Check sheet for the modelled part. Datum: model origin and axes. Units: mm. Round coordinates to 2 decimals unless told otherwise and drop trailing zeros. Order: outer loops, then holes, each group sorted by start corner. A loop starts at its lowest first (then second) coordinate and runs counter-clockwise, first axis right, second up.
Q1. Cross-section at C-C on y = 5. Record the cut outline in (x, z).
Q2. Cross-section at D-D on z = 0.55. Give the number of separate pieces and of enclosed holes in the cut face, then the cut area to 3 significant figures.
Q3. Depth check by flat-ended pin: P1, Ø2.5, axis at x = -53.03, y = -53.03, coming from the +Z side. Enter the tip coordinate at first touch or a pass-through.
Q4. Cross-section at A-A on x = 0. Record the cut outline in (y, z), then the cut area to 3 significant figures.
Q5. Cross-section at B-B on y = -23. Record the cut outline in (x, z), then the cut area to 3 significant figures.
Q6. Scan lines: probe 1 along X at (y, z) = (-43, 0.8); probe 2 along Y at (x, z) = (53, 2.3); probe 3 along Y at (x, z) = (-17, 2.3). Record each from-to range of solid material in increasing order.
from build123d import *

# Parameters (mm, degrees)
SKETCH_1_W      = 140
SKETCH_1_H      = 140
SKETCH_1_R      = 1.6
SKETCH_1_R_2    = 1.1
SKETCH_1_R_3    = 15
EXTRUDE_1_DEPTH = 3
FILLET_1_R      = 5


with BuildPart() as part:
    # 草图1 → 凸台-拉伸1 (new body)
    with BuildSketch(Plane.XY):
        Rectangle(SKETCH_1_W, SKETCH_1_H)
        with Locations((53.033008589, 53.033008589)):
            Circle(SKETCH_1_R, mode=Mode.SUBTRACT)
        with Locations((-29, 43)):
            Circle(SKETCH_1_R_2, mode=Mode.SUBTRACT)
        with Locations((29, 43)):
            Circle(SKETCH_1_R_2, mode=Mode.SUBTRACT)
        with Locations(Location((29, -43, 0), (0, 0, 180))):
            Circle(SKETCH_1_R_2, mode=Mode.SUBTRACT)
        with Locations(Location((-29, -43, 0), (0, 0, 180))):
            Circle(SKETCH_1_R_2, mode=Mode.SUBTRACT)
        with Locations((53.033008589, -53.033008589)):
            Circle(SKETCH_1_R, mode=Mode.SUBTRACT)
        with Locations((-53.033008589, -53.033008589)):
            Circle(SKETCH_1_R, mode=Mode.SUBTRACT)
        with Locations((-53.033008589, 53.033008589)):
            Circle(SKETCH_1_R, mode=Mode.SUBTRACT)
        with Locations((45.961940777, 45.961940777)):
            Circle(SKETCH_1_R, mode=Mode.SUBTRACT)
        with Locations((38.890872965, 38.890872965)):
            Circle(SKETCH_1_R, mode=Mode.SUBTRACT)
        with Locations((45.961940777, -45.961940777)):
            Circle(SKETCH_1_R, mode=Mode.SUBTRACT)
        with Locations((38.890872965, -38.890872965)):
            Circle(SKETCH_1_R, mode=Mode.SUBTRACT)
        with Locations((-45.961940777, -45.961940777)):
            Circle(SKETCH_1_R, mode=Mode.SUBTRACT)
        with Locations((-38.890872965, -38.890872965)):
            Circle(SKETCH_1_R, mode=Mode.SUBTRACT)
        with Locations((-45.961940777, 45.961940777)):
            Circle(SKETCH_1_R, mode=Mode.SUBTRACT)
        with Locations((-38.890872965, 38.890872965)):
            Circle(SKETCH_1_R, mode=Mode.SUBTRACT)
        Circle(SKETCH_1_R_3, mode=Mode.SUBTRACT)
        with BuildLine():
            Line((-25, 58.033008589), (25, 58.033008589))
            ThreePointArc((25, 58.033008589), (30, 53.033008589), (25, 48.033008589))
            Line((25, 48.033008589), (-25, 48.033008589))
            ThreePointArc((-25, 48.033008589), (-30, 53.033008589), (-25, 58.033008589))
        make_face(mode=Mode.SUBTRACT)
        with BuildLine():
            Line((58.033008589, 25), (58.033008589, -25))
            ThreePointArc((58.033008589, -25), (53.033008589, -30), (48.033008589, -25))
            Line((48.033008589, -25), (48.033008589, 25))
            ThreePointArc((48.033008589, 25), (53.033008589, 30), (58.033008589, 25))
        make_face(mode=Mode.SUBTRACT)
        with BuildLine():
            Line((25, -58.033008589), (-25, -58.033008589))
            ThreePointArc((-25, -58.033008589), (-30, -53.033008589), (-25, -48.033008589))
            Line((-25, -48.033008589), (25, -48.033008589))
            ThreePointArc((25, -48.033008589), (30, -53.033008589), (25, -58.033008589))
        make_face(mode=Mode.SUBTRACT)
        with BuildLine():
            Line((-58.033008589, -25), (-58.033008589, 25))
            ThreePointArc((-58.033008589, 25), (-53.033008589, 30), (-48.033008589, 25))
            Line((-48.033008589, 25), (-48.033008589, -25))
            ThreePointArc((-48.033008589, -25), (-53.033008589, -30), (-58.033008589, -25))
        make_face(mode=Mode.SUBTRACT)
    extrude(amount=EXTRUDE_1_DEPTH)

    # 圆角1
    fillet_1_edges = [part.edges().sort_by_distance(p)[0] for p in [
        (-70, 70, 1.5),
        (70, 70, 1.5),
        (70, -70, 1.5),
        (-70, -70, 1.5),
    ]]
    fillet(fillet_1_edges, radius=FILLET_1_R)


solid = part.part
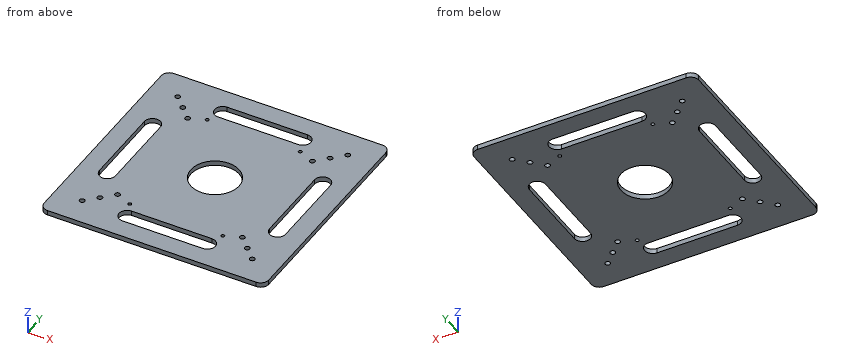
Results found:
1. outline: (-70, 0) - (-58.03, 0) - (-58.03, 3) - (-70, 3) - close; (-48.03, 0) - (-14.14, 0) - (-14.14, 3) - (-48.03, 3) - close; (14.14, 0) - (48.03, 0) - (48.03, 3) - (14.14, 3) - close; (58.03, 0) - (70, 0) - (70, 3) - (58.03, 3) - close
2. separate pieces: 1
2. enclosed holes: 21
2. area: 16,400 mm2
3. P1: passes through
4. outline: (-70, 0) - (-58.03, 0) - (-58.03, 3) - (-70, 3) - close; (-48.03, 0) - (-15, 0) - (-15, 3) - (-48.03, 3) - close; (15, 0) - (48.03, 0) - (48.03, 3) - (15, 3) - close; (58.03, 0) - (70, 0) - (70, 3) - (58.03, 3) - close
4. area: 270 mm2
5. outline: (-70, 0) - (-58.03, 0) - (-58.03, 3) - (-70, 3) - close; (-48.03, 0) - (48.03, 0) - (48.03, 3) - (-48.03, 3) - close; (58.03, 0) - (70, 0) - (70, 3) - (58.03, 3) - close
5. area: 360 mm2
6. probe 1: x = -70 to -30.1, -27.9 to 27.9, 30.1 to 70
6. probe 2: y = -70 to -54.63, -51.43 to -30, 30 to 51.43, 54.63 to 70
6. probe 3: y = -70 to -58.03, -48.03 to 48.03, 58.03 to 70
